from build123d import *

# Parameters (mm, degrees)
BOSS_EXTRUDE2_DEPTH                                = 110
CHAMBRAGE_POUR_VIS_T_TE_RONDE_BOMB_E_M_D           = 3.4
CHAMBRAGE_POUR_VIS_T_TE_RONDE_BOMB_E_M_DEPTH       = 7
CHAMBRAGE_POUR_VIS_T_TE_RONDE_BOMB_E_M_CBORE_D     = 7
CHAMBRAGE_POUR_VIS_T_TE_RONDE_BOMB_E_M_CBORE_DEPTH = 2.4
CUT_EXTRUDE1_DEPTH                                 = 111.147379253
CHAMFER1_SIZE                                      = 0.3


with BuildPart() as part:
    # Sketch1 → Boss-Extrude2 (new body)
    with BuildSketch(Plane.XY):
        Polygon((-1.8125, 5.4), (-0.8125, 5.4), (1.8125, 2.775), (1.8125, -2.775), (-0.8125, -5.4), (-1.8125, -5.4), align=None)
    extrude(amount=BOSS_EXTRUDE2_DEPTH)

    # Chambrage pour vis _ t_te ronde bomb_e M
    with Locations(Plane.ZY.offset(1.8125)):
        with Locations((60, 0), (50, 0), (38, 0), (26, 0), (14, 0), (72, 0), (84, 0), (96, 0)):
            CounterBoreHole(CHAMBRAGE_POUR_VIS_T_TE_RONDE_BOMB_E_M_D / 2, CHAMBRAGE_POUR_VIS_T_TE_RONDE_BOMB_E_M_CBORE_D / 2, CHAMBRAGE_POUR_VIS_T_TE_RONDE_BOMB_E_M_CBORE_DEPTH, depth=CHAMBRAGE_POUR_VIS_T_TE_RONDE_BOMB_E_M_DEPTH)

    # Sketch2 → Cut-Extrude1 (cut, through all)
    with BuildSketch(Plane.XY.offset(110)):
        Polygon((-0.8125, 5.4), (-1.8125, 4.4), (-1.8125, 5.4), align=None)
        Polygon((-0.8125, -5.4), (-1.8125, -4.4), (-1.8125, -5.4), align=None)
    extrude(amount=-CUT_EXTRUDE1_DEPTH, mode=Mode.SUBTRACT)

    # Chamfer1
    chamfer1_edges = [part.edges().sort_by_distance(p)[0] for p in [
        (-0.8125, 5.4, 55),
        (-0.8125, -5.4, 55),
    ]]
    chamfer(chamfer1_edges, length=CHAMFER1_SIZE)


solid = part.part
Could you check a few things on this model? Use its own coordinates, in mm. A direction names the side the tool comes from. Give positions to 0.01 mm unless a question says otherwise; leave off trailing zeros. Order: outer loops, then holes, each group sorted by start corner. A loop starts at its lowest first (then second) coordinate and runs counter-clockwise, first axis right, second up. Notation, with made-up numbers: (48.5, 85) - (92.5, 85) arc R30 ccw to (92.5, 120) - close; hole circle Ø4 at (-29, 68). An arc over 180 degrees is marked (long way). Return JSON: item names as keys, results as strings. Group by question number.
Q1. Please list where these lines run through material, in increasing order: line 1 along Y through (x, z) = (0.15, 60); line 2 along X through (y, z) = (2.5, 97); line 3 along X through (y, z) = (4, 75.5). Write a range as [from, to].
Q2. Will these pins go through, and if not, where does the flat tip stop? pin 1 Ø5.5 at (y, z) = (0.5, 25.5) entering from -X; pin 2 Ø3.5 at (y, z) = (-1.5, 70.5) entering from -X.
Q3. Suppose I cut it at A-A, the plane z = 38. Please give me the cut outline in (x, y) (1 decimal), and give its area (3 significant figures).
Q4. Suppose I cut it at D-D, the plane z = 25.5. Please give me the cut outline in (x, y) (1 decimal).
Q5. Which directions (+Z, -Z, +X, -X, +Y, -Y) give clear straight access to the entire face, cutting with the end or side of a thin tool? Please do faces 5 (the face through (1.21, 0.07, 85.7)), 6 (the face through (0.587, -2, 25)).
Q6. Thinking about a two-plate mould opening in Z: for faces 1 (the face through (-1.812, 0, 54)), 2 (the face through (1.21, 0.07, 97.7)), 3 (the face through (0, 0, 0)), 4 (the face through (0, 0, 110)), which applies, pulls with the +Z half, pulls with the -Z half, needs draft (parallel to the pull), parting line crosses it, or undercut?
Q7. Suppose I cut it at B-B, the plane x = 1.2. State how many separate pieces and enclosed holes the cut face has, and give its area (3 significant figures).
Resolved:
{
 "1": {"line 1": "y = [-4.44, -3.5], [3.5, 4.44]", "line 2": "x = [0.59, 1.81]", "line 3": "x = [-1.81, 0.59]"},
 "2": {"pin 1": "stops at x = 0.59", "pin 2": "stops at x = -1.81"},
 "3": {"outline": "(-1.8, -4.4) - (-1, -5.2) - (-0.6, -5.2) - (1.8, -2.8) - (1.8, -1.7) - (0.6, -1.7) - (0.6, -3.5) - (-1.8, -3.5) - close; (-1.8, 3.5) - (0.6, 3.5) - (0.6, 1.7) - (1.8, 1.7) - (1.8, 2.8) - (-0.6, 5.2) - (-1, 5.2) - (-1.8, 4.4) - close", "area": "10.2 mm2"},
 "4": {"outline": "(-1.8, -4.4) - (-1, -5.2) - (-0.6, -5.2) - (1.8, -2.8) - (1.8, -1.6) - (0.6, -1.6) - (0.6, -3.5) - (-1.8, -3.5) - close; (-1.8, 3.5) - (0.6, 3.5) - (0.6, 1.6) - (1.8, 1.6) - (1.8, 2.8) - (-0.6, 5.2) - (-1, 5.2) - (-1.8, 4.4) - close"},
 "5": {"face 5": "+X, -X", "face 6": "-X"},
 "6": {"face 1": "needs draft", "face 2": "undercut", "face 3": "pulls with the -Z half", "face 4": "pulls with the +Z half"},
 "7": {"separate pieces": "1", "enclosed holes": "8", "area": "673 mm2"}
}
